```python
from build123d import *

# Parameters (mm, degrees)
F1_DEPTH = 41.425
F2_R     = 1.55
F3_DEPTH = 22.339877


with BuildPart() as f1:
    # F0 (on Front) → F1 (new body, symmetric)
    with BuildSketch(Plane.XZ):
        Polygon((-22.752756, 18.288877), (-60.822756, 18.288877), (-60.822756, 7.558877), (-22.752756, 7.558877), (-22.625374, 9.708877), (38.016342, 9.708877), (37.817244, 7.578877), (75.887244, 7.578877), (75.887244, 18.288877), (37.817244, 18.288877), (37.817244, 22.338877), (-22.752756, 22.338877), align=None)
    extrude(amount=F1_DEPTH, both=True)

    # F2 (on Top) → F3 (cut, through all)
    with BuildSketch(Plane.XY):
        with Locations((-48.862756, 30.375)):
            Circle(F2_R)
        with Locations((63.927244, 27.275)):
            Circle(F2_R)
        with Locations((63.927244, -27.275)):
            Circle(F2_R)
        with Locations((-48.862756, -27.275)):
            Circle(F2_R)
    extrude(amount=F3_DEPTH, mode=Mode.SUBTRACT)


solid = f1.part
```
Input: part model. Units: mm. Frame: model coordinates. A direction names the side the tool comes from. Give positions to 0.01 mm unless a question says otherwise; leave off trailing zeros. Order: outer loops, then holes, each group sorted by start corner. A loop starts at its lowest first (then second) coordinate and runs counter-clockwise, first axis right, second up. Notation, with made-up numbers: (65, 79) - (72, 79) arc R8 cw to (72, 90) - close; hole circle Ø5 at (32, 10.5). An arc over 180 degrees is marked (long way). Put each result on its own line as item: value.
Item 1: Contact query for flat-ended pins moving along their axis: pin 1 (1 mm diameter, centred on x = -22, y = -10, fed in from -Z); pin 2 (4 mm diameter, centred on x = 60, y = 28.5, fed in from +Z); pin 3 (1.2 mm diameter, centred on y = 2.5, z = 21, fed in from -X). Output: stop coordinate, or through.
Found:
pin 1: stops at z = 9.71
pin 2: stops at z = 18.29
pin 3: stops at x = -22.75
Item 2: Draft query along Y for faces 3 (the flat face through (7, 41.425, 15)), 4 (the flat face through (57, -1, 18.289)), 5 (the cylindrical face through (65.406, 27.741, 12.859)), 6 (the flat face through (7, -41.425, 15)). Return one class per face: +Y half, -Y half, draft (parallel to the pull), parting line (faces both ways), or undercut.
Found:
face 3: +Y half
face 4: draft
face 5: undercut
face 6: -Y half
Item 3: Section query C-C, the plane x = 48.5. Return loops of the section in (y, z) (3 decimals).
Found:
outline: (-41.425, 7.579) - (41.425, 7.579) - (41.425, 18.289) - (-41.425, 18.289) - close
Item 4: Ray query, L1, parallel to Z at x = 6.5, y = -7; L2, parallel to Z at x = -48, y = -14; L3, parallel to X at y = 28.5, z = 10.5. Return the intervals inside material, ascending. Write a range as from..to.
Found:
L1: z = 9.71..22.34
L2: z = 7.56..18.29
L3: x = -60.82..62.98, 64.88..75.89
Item 5: Access query for faces 1 (the flat face through (37.817, -1, 20)), 2 (the flat face through (-22.753, -1, 20)). Directions: +Z, -Z, +X, -X, +Y, -Y. A direction counts if a zero-diameter tool reaches every point of the face in a straight line with its end or side. Return the directions, or none.
Found:
face 1: +Z, +X, +Y, -Y
face 2: +Z, -X, +Y, -Y
Item 6: Section query A-A, the plane y = 0.5. Return loops of the section in (x, z), then the cut area to 3 significant figures.
Found:
outline: (-60.82, 7.56) - (-22.75, 7.56) - (-22.63, 9.71) - (38.02, 9.71) - (37.82, 7.58) - (75.89, 7.58) - (75.89, 18.29) - (37.82, 18.29) - (37.82, 22.34) - (-22.75, 22.34) - (-22.75, 18.29) - (-60.82, 18.29) - close
area: 1,580 mm^2
Item 7: Section query B-B, the plane x = 6. Return loops of the section in (y, z) (3 decimals), then the cut area to 3 significant figures.
Found:
outline: (-41.425, 9.709) - (41.425, 9.709) - (41.425, 22.339) - (-41.425, 22.339) - close
area: 1,050 mm^2
